```python
from build123d import *

# Parameters (mm, degrees)
BOSS_EXTRUDE7_DEPTH = 80
FILLET1_R           = 10
FILLET2_R           = 10
SKETCH3_W           = 20
SKETCH3_H           = 28.966426772
CUT_EXTRUDE1_DEPTH  = 40
FILLET4_R           = 20


with BuildPart() as part:
    # Sketch2 → Boss-Extrude7 (new body)
    with BuildSketch(Plane(origin=(0, 0, 0), x_dir=(0, 0, -1), z_dir=(1, 0, 0))):
        with BuildLine():
            ThreePointArc((-1.339745962, 10), (-19.659258263, 17.588190451), (0, 15))
            Line((0, 15), (10, 15))
            ThreePointArc((10, 15), (-28.228756555, 23.228756555), (3.228756555, 0))
            Line((3.228756555, 0), (90, 0))
            Line((90, 0), (100, 0))
            Line((100, 0), (100, 10))
            Line((100, 10), (100, 31))
            Line((100, 31), (90, 31))
            Line((90, 31), (90, 10))
            Line((90, 10), (20, 10))
            Line((20, 10), (10, 10))
            Line((10, 10), (-1.339745962, 10))
        make_face()
    extrude(amount=BOSS_EXTRUDE7_DEPTH)

    # Fillet1
    fillet1_edges = [part.edges().sort_by_distance(p)[0] for p in [
        (40, 10, -90),
    ]]
    fillet(fillet1_edges, radius=FILLET1_R)

    # Fillet2
    fillet2_edges = [part.edges().sort_by_distance(p)[0] for p in [
        (40, 10, 1.339745962),
        (40, 0, -3.228756555),
    ]]
    fillet(fillet2_edges, radius=FILLET2_R)

    # Sketch3 → Cut-Extrude1 (cut, symmetric)
    with BuildSketch(Plane(origin=(0, 0, 0), x_dir=(1, 0, 0), z_dir=(0, 1, 0))):
        with BuildLine():
            Line((53, 10), (53, 23.645843496))
            ThreePointArc((53, 23.645843496), (40, 70), (27, 23.645843496))
            Line((27, 23.645843496), (27, 10))
            Line((27, 10), (27, -31.662975448))
            Line((27, -31.662975448), (53, -31.662975448))
            Line((53, -31.662975448), (53, 10))
        make_face()
        with Locations((40, 94.483213386)):
            Rectangle(SKETCH3_W, SKETCH3_H)
    extrude(amount=CUT_EXTRUDE1_DEPTH, both=True, mode=Mode.SUBTRACT)

    # Fillet4
    fillet4_edges = [part.edges().sort_by_distance(p)[0] for p in [
        (15, 0, -100),
        (65, 0, -100),
    ]]
    fillet(fillet4_edges, radius=FILLET4_R)


solid = part.part
```
Check sheet for the modelled part. Datum: model origin and axes. Units: mm. A direction names the side the tool comes from. Coordinates: 2 decimals unless noted, no trailing zeros. Loops run counter-clockwise (first coordinate to the right, second up) from the corner with the lowest first, then second, coordinate; pieces in that order, holes last. Notation, with made-up numbers: M -39.5,31.5 L -32.5,31.5 A16 ccw -32.5,35.5 Z; hole C 35.25,66.25 d9. An arc over 180 degrees is marked long. Answer as a JSON object with one key per item and string values.
1. Release check for a two-part mould opening along Z. For faces 1 (the flat face through (15, 26, -90)), 2 (the cylindrical face through (65.21, 5.703, -93.986)), 3 (the flat face through (15, 31, -95)), 4 (the cylindrical face through (13.311, 25.104, 27.26)) record: pulls with the +Z half, pulls with the -Z half, needs draft (parallel to the pull), parting line crosses it, or undercut.
Outcome:
{"face 1": "undercut", "face 2": "pulls with the -Z half", "face 3": "needs draft", "face 4": "undercut"}
2. Scan lines: L1, parallel to Y at x = 66.5, z = 10; L2, parallel to Z at x = 70.5, y = 17; L3, parallel to X at y = -3, z = 9.5. Record each from-to range of solid material in increasing order. Write a range as from..to.
Outcome:
{"L1": "-5..5, 25..35", "L2": "-99.77..-89.54, -9.9..0.2, 19.8..29.9", "L3": "0..27, 53..80"}
3. Sectioned sample at C-C on z = -45. Record the cut outline in (x, y), and give its area (3 significant figures).
Outcome:
{"outline": "M 0,0 L 15,0 L 15,10 L 0,10 Z; M 65,0 L 80,0 L 80,10 L 65,10 Z", "area": "300 mm²"}
4. Sectioned sample at B-B on y = 17.5. Record the cut outline in (x, z), and give its area (3 significant figures).
Outcome:
{"outline": "M 0,-99.84 L 30,-99.84 L 30,-89.68 L 0,-89.68 Z; M 0,-9.84 L 27,-9.84 L 27,0.32 L 0,0.32 Z; M 0,19.68 L 27,19.68 L 27,29.84 L 0,29.84 Z; M 50,-99.84 L 80,-99.84 L 80,-89.68 L 50,-89.68 Z; M 53,-9.84 L 80,-9.84 L 80,0.32 L 53,0.32 Z; M 53,19.68 L 80,19.68 L 80,29.84 L 53,29.84 Z", "area": "1,710 mm²"}
5. Access from +Z, -Z, +X, -X, +Y, -Y to the whole of each face (thin tool, end or side, straight path). Record for faces 5 (the flat face through (50, 16, -92)), 6 (the cylindrical face through (15.21, 13.01, -87.15)), 7 (the flat face through (22, 0, -26)), 8 (the flat face through (53, 6, 4)), 9 (the flat face through (66, 15, -5)).
Outcome:
{"face 5": "-Z, +Y, -Y", "face 6": "+X, -X, +Y", "face 7": "-Z, +X, -X, -Y", "face 8": "+Z, +Y, -Y", "face 9": "+X, -X"}
6. Sectioned sample at A-A on z = 10. Record the cut outline in (x, y).
Outcome:
{"outline": "M 0,-5 L 27,-5 L 27,5 L 0,5 Z; M 0,25 L 27,25 L 27,35 L 0,35 Z; M 53,-5 L 80,-5 L 80,5 L 53,5 Z; M 53,25 L 80,25 L 80,35 L 53,35 Z"}
7. Sectioned sample at D-D on x = 13. Record the cut outline in (y, z), and give its area (3 significant figures).
Outcome:
{"outline": "M -1.67,-1.06 A10 cw 0,-6.58 L 0,-80 A20 ccw 20,-100 L 31,-100 L 31,-90 L 20,-90 A10 cw 10,-80 L 10,-3.23 A10 ccw 7.5,3.39 A10 cw long 15,0 L 15,-10 A20 ccw long Z", "area": "1,970 mm²"}
8. Depth check by flat-ended pin: P1, Ø5, axis at x = 58, z = -93.5, coming from the +Y side; P2, Ø2, axis at x = 27.5, y = 18.5, coming from the -Z side; P3, Ø5, axis at x = 69, z = -14.5, coming from the +Y side; P4, Ø16, axis at y = 16, z = -93, coming from the -X side. Enter the tip coordinate at first touch or a pass-through.
Outcome:
{"P1": "y = 31", "P2": "z = -99.99", "P3": "y = 10", "P4": "x = 0"}
